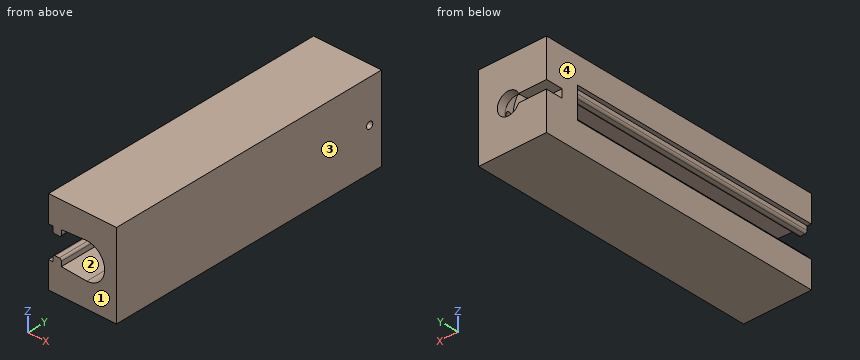
from build123d import *

# Parameters (mm, degrees)
SKETCH5_W           = 4
SKETCH5_H           = 5
BOSS_EXTRUDE3_DEPTH = 15
CUT_EXTRUDE1_DEPTH  = 16.37245914
FILLET1_R           = 0.125
SKETCH6_W           = 4
SKETCH6_H           = 5
SKETCH6_R           = 0.425
BOSS_EXTRUDE4_DEPTH = 1
SKETCH7_W           = 4
SKETCH7_H           = 5
SKETCH7_RX          = 1.3
SKETCH7_RY          = 0.65
BOSS_EXTRUDE5_DEPTH = 0.5
SKETCH9_W           = 4
SKETCH9_H           = 5
SKETCH9_R           = 0.65
BOSS_EXTRUDE6_DEPTH = 0.5
CUT_EXTRUDE2_REACH  = 19.33
SKETCH10_W          = 1.65
SKETCH10_H          = 0.5
CUT_EXTRUDE3_REACH  = 19.642
SKETCH11_R          = 0.2


with BuildPart() as part:
    # Sketch5 → Boss-Extrude3 (new body)
    with BuildSketch(Plane(origin=(0, 0, 0), x_dir=(1, 0, 0), z_dir=(0, 1, 0))):
        with Locations((-0.25, 0)):
            Rectangle(SKETCH5_W, SKETCH5_H)
    extrude(amount=BOSS_EXTRUDE3_DEPTH)

    # Sketch3 → Cut-Extrude1 (cut, through all)
    with BuildSketch(Plane(origin=(0, 0, 0), x_dir=(1, 0, 0), z_dir=(0, 1, 0))):
        with BuildLine():
            Line((-2.5, 0.9), (-2, 0.93))
            Line((-2, 0.93), (-2, 0.56))
            Line((-2, 0.56), (-1.5, 0.56))
            Line((-1.5, 0.56), (-1.5, 0.96))
            Line((-1.5, 0.96), (0, 1.05))
            ThreePointArc((0, 1.05), (1.05, 0), (0, -1.05))
            Line((0, -1.05), (-1.5, -0.96))
            Line((-1.5, -0.96), (-1.5, -0.56))
            Line((-1.5, -0.56), (-2, -0.56))
            Line((-2, -0.56), (-2, -0.93))
            Line((-2, -0.93), (-2.5, -0.9))
            Line((-2.5, -0.9), (-5, -0.9))
            ThreePointArc((-5, -0.9), (-5.9, 0), (-5, 0.9))
            Line((-5, 0.9), (-2.5, 0.9))
        make_face()
    extrude(amount=CUT_EXTRUDE1_DEPTH, mode=Mode.SUBTRACT)

    # Fillet1
    fillet1_edges = [part.edges().sort_by_distance(p)[0] for p in [
        (-1.5, 7.5, -0.56),
        (-2, 7.5, -0.56),
        (-2, 7.5, 0.56),
        (-1.5, 7.5, 0.56),
    ]]
    fillet(fillet1_edges, radius=FILLET1_R)

    # Sketch6 → Boss-Extrude4 (add)
    with BuildSketch(Plane(origin=(0, 15, 0), x_dir=(1, 0, 0), z_dir=(0, 1, 0))):
        with Locations((-0.25, 0)):
            Rectangle(SKETCH6_W, SKETCH6_H)
        with Locations(Location((0, 0, 0), (0, 0, 270))):
            Circle(SKETCH6_R, mode=Mode.SUBTRACT)
    extrude(amount=BOSS_EXTRUDE4_DEPTH)

    # Sketch7 → Boss-Extrude5 (add)
    with BuildSketch(Plane(origin=(0, 16, 0), x_dir=(1, 0, 0), z_dir=(0, 1, 0))):
        with Locations((-0.25, 0)):
            Rectangle(SKETCH7_W, SKETCH7_H)
        with Locations(Location((0, 0), (0, 0, 90))):
            Ellipse(SKETCH7_RX, SKETCH7_RY, mode=Mode.SUBTRACT)
    extrude(amount=BOSS_EXTRUDE5_DEPTH)

    # Sketch9 → Boss-Extrude6 (add)
    with BuildSketch(Plane(origin=(0, 16.5, 0), x_dir=(1, 0, 0), z_dir=(0, 1, 0))):
        with Locations((-0.25, 0)):
            Rectangle(SKETCH9_W, SKETCH9_H)
        Circle(SKETCH9_R, mode=Mode.SUBTRACT)
    extrude(amount=BOSS_EXTRUDE6_DEPTH)

    # Cut-Extrude2: up to this face of the body (flat: up to its plane)
    cut_extrude2_end = Plane(part.part.faces().sort_by_distance((0.0037652, 16, 1.270907163))[0])
    # Sketch10 → Cut-Extrude2 (cut, up to the picked face)
    with BuildSketch(Plane(origin=(0, 17, 0), x_dir=(1, 0, 0), z_dir=(0, 1, 0)), mode=Mode.PRIVATE) as cut_extrude2_sk1:
        with Locations((-1.425, 0)):
            Rectangle(SKETCH10_W, SKETCH10_H)
    cut_extrude2_tool1 = split(extrude(cut_extrude2_sk1.sketch, amount=-CUT_EXTRUDE2_REACH, mode=Mode.PRIVATE), bisect_by=cut_extrude2_end, keep=Keep.BOTH, mode=Mode.PRIVATE)
    add(cut_extrude2_tool1.solids().sort_by(Axis((-1.425, 17, 0), (0, -1, 0)))[0], mode=Mode.SUBTRACT)

    # Sketch11 → Cut-Extrude3 (cut, up to next)
    with BuildSketch(Plane(origin=(1.75, 0, 0), x_dir=(0, 0, -1), z_dir=(1, 0, 0)), mode=Mode.PRIVATE) as cut_extrude3_sk1:
        with Locations((0, 16.25)):
            Circle(SKETCH11_R)
    cut_extrude3_tool1 = extrude(cut_extrude3_sk1.sketch, amount=-CUT_EXTRUDE3_REACH, mode=Mode.PRIVATE) & part.part
    add(cut_extrude3_tool1.solids().sort_by_distance((1.75, 16.25, 0))[0], mode=Mode.SUBTRACT)


solid = part.part
Here's how the part is built. I have some questions about the finished solid (model axes, mm). Face numbers are marked on the shaded views. Round coordinates to 2 decimals unless told otherwise and drop trailing zeros. Order: outer loops, then holes, each group sorted by start corner. A loop starts at its lowest first (then second) coordinate and runs counter-clockwise, first axis right, second up. Notation, with made-up numbers: (27, 82) -> (50, 82) arc R30 cw to (50, 105) -> close; hole circle Ø9 at (76.25, -17.5). An arc over 180 degrees is marked (long way). Return JSON: item names as keys, results as strings.
Q1. If we mould it in two halves opening along X, with no side actions, what happens to the marked faces 1, 2, 3 and 4? For each: released by +X, released by -X, zero draft, split by the parting line, or undercut.
Filled sheet:
{"face 1": "zero draft", "face 2": "undercut", "face 3": "released by +X", "face 4": "released by -X"}
Q2. If we section it at B-B on x = -1.05: List the corners of the cut face in (y, z) for me.
Filled sheet:
{"outline": "(0, -2.5) -> (17, -2.5) -> (17, -0.25) -> (16, -0.25) -> (16, 0.25) -> (17, 0.25) -> (17, 2.5) -> (0, 2.5) -> (0, 0.99) -> (15, 0.99) -> (15, -0.99) -> (0, -0.99) -> close"}
Q3. I need wall thicknesses on line 1 along Y through (x, z) = (1.45, 0); line 2 along X through (y, z) = (15.4, 0) (3 decimals); line 3 along Z through (x, y) = (1, 16.25). Which ranges of each line are inside material? Lowest first, please. Write a range as from..to.
Filled sheet:
{"line 1": "y = 0..16.05, 16.45..17", "line 2": "x = -2.25..-0.425, 0.425..1.75", "line 3": "z = -2.5..-0.2, 0.2..2.5"}
Q4. For pin 1 Ø1.2 at (x, z) = (0, 0) entering from +Y, with a flat end and sliding along its axis, tell me the tip position at first contact or that it passes through.
Filled sheet:
{"pin 1": "stops at y = 16"}
Q5. If we section it at A-A on y = 13.5: List the corners of the cut face in (x, z) for me (3 decimals).
Filled sheet:
{"outline": "(-2.25, -2.5) -> (1.75, -2.5) -> (1.75, 2.5) -> (-2.25, 2.5) -> (-2.25, 0.915) -> (-2, 0.93) -> (-2, 0.685) arc R0.125 ccw to (-1.875, 0.56) -> (-1.625, 0.56) arc R0.125 ccw to (-1.5, 0.685) -> (-1.5, 0.96) -> (0, 1.05) arc R1.05 cw to (0, -1.05) -> (-1.5, -0.96) -> (-1.5, -0.685) arc R0.125 ccw to (-1.625, -0.56) -> (-1.875, -0.56) arc R0.125 ccw to (-2, -0.685) -> (-2, -0.93) -> (-2.25, -0.915) -> close"}
